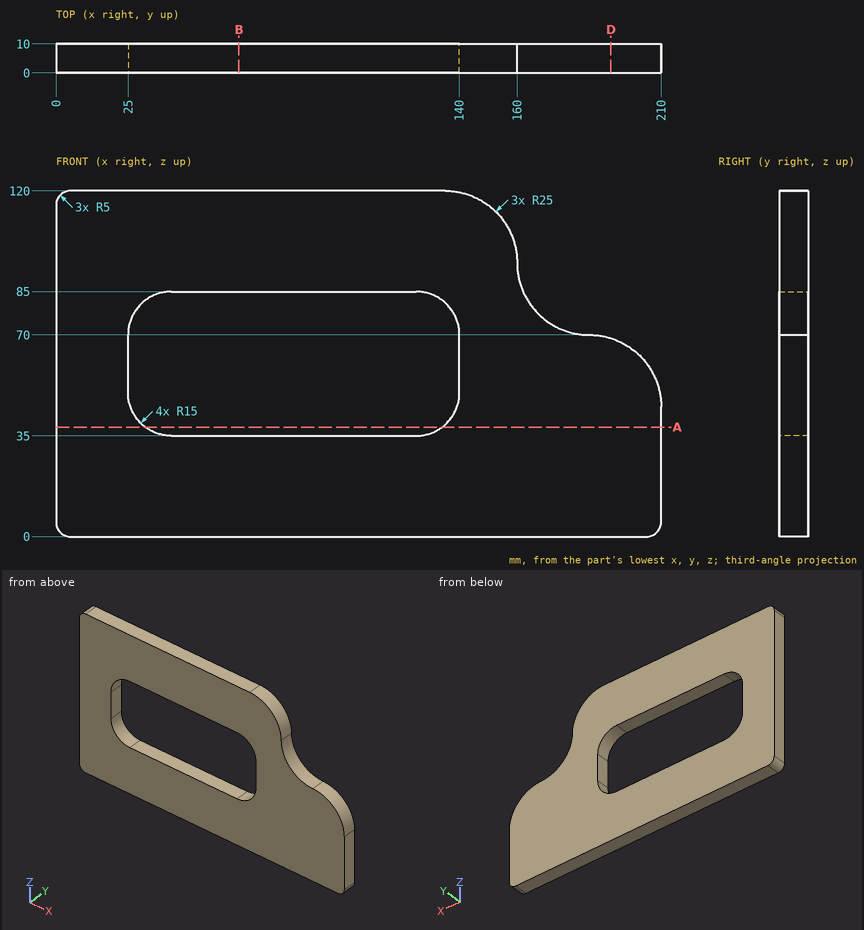
Part print with two shaded views. Sizes in mm from the minimum x, y, z corner. Round coordinates to 2 decimals unless told otherwise and drop trailing zeros. Write each loop counter-clockwise with the first axis right and the second up, starting at its lowest first coordinate (ties: lowest second). Pieces come first, ordered by that corner, then holes. Notation, with made-up numbers: (38, -29.5) - (52, -29.5) arc R15 ccw to (52, -11.5) - close; hole circle Ø7 at (53, 15). An arc over 180 degrees is marked (long way). Answer as CSV lines item,"result".
Q1. Drop flat-ended pins along their axis: pin 1 (1 mm diameter, centred on x = 178, y = 7, fed in from +Z); pin 2 (1.5 mm diameter, centred on x = 100.5, z = 15, fed in from -Y). Give the stop position or say it passes through.
Report:
pin 1,"stops at z = 71.15"
pin 2,"stops at y = 0"
Q2. Drill centre lines: probe 1 along Z at (x, y) = (60, 2); probe 2 along Z at (x, y) = (131, 3.25); probe 3 along X at (y, z) = (5, 96.5). Where is each one in solid material? Low to high. Write a range as [from, to].
Report:
probe 1,"z = [0, 35], [85, 120]"
probe 2,"z = [0, 36.25], [83.75, 120]"
probe 3,"x = [0, 159.95]"
Q3. Cut at A-A (z = 38). Write the cut outline in (x, y).
Report:
outline,"(0, 0) - (31, 0) - (31, 10) - (0, 10) - close; (134, 0) - (210, 0) - (210, 10) - (134, 10) - close"
Q4. Cut at D-D (x = 192.5). Write the cut outline in (y, z).
Report:
outline,"(0, 0) - (10, 0) - (10, 68.85) - (0, 68.85) - close"
Q5. Cut at B-B (x = 63.5). Write the cut outline in (y, z).
Report:
outline,"(0, 0) - (10, 0) - (10, 35) - (0, 35) - close; (0, 85) - (10, 85) - (10, 120) - (0, 120) - close"
